from build123d import *

# Parameters (mm, degrees)
CHAMFER1_SIZE       = 1
SKETCH2_R           = 2.5
BOSS_EXTRUDE1_DEPTH = 1


with BuildPart() as part:
    # Sketch1 → Revolve1 (revolve)
    with BuildSketch(Plane.XY, mode=Mode.PRIVATE) as revolve1_sk:
        Polygon((0, 25), (-5, 25), (-5, 23), (-2.5, 23), (-2.5, 22), (-2, 22), (-2, 0), (-0.45, 0), (-0.45, 19), (0, 19), align=None)
    revolve(revolve1_sk.sketch.rotate(Axis((0, 0, 0), (0, 1, 0)), 270), axis=Axis((0, 0, 0), (0, 1, 0)))

    # Chamfer1
    chamfer1_edges = [part.edges().sort_by_distance(p)[0] for p in [
        (0, 0, 2),
    ]]
    chamfer(chamfer1_edges, length=CHAMFER1_SIZE)

    # Sketch2 → Boss-Extrude1 (add)
    with BuildSketch(Plane(origin=(0, 25, 0), x_dir=(1, 0, 0), z_dir=(0, 1, 0))):
        with Locations(Location((0, 0, 0), (0, 0, 90))):
            Circle(SKETCH2_R)
    extrude(amount=BOSS_EXTRUDE1_DEPTH)


solid = part.part
Here's how the part is built. I have some questions about the finished solid (model axes, mm). A direction names the side the tool comes from. Coordinates: 2 decimals unless noted, no trailing zeros. Write each loop counter-clockwise with the first axis right and the second up, starting at its lowest first coordinate (ties: lowest second). Pieces come first, ordered by that corner, then holes.
1) If I drill on line 1 (X direction, y = 13, z = 0); line 2 (Y direction, x = 1.5, z = 3); line 3 (Z direction, x = 0.25, y = 11.75), over which ranges is the centre line in solid material (lowest first)?
Filled in:
line 1: x = -2 to -0.45, 0.45 to 2
line 2: y = 23 to 25
line 3: z = -1.98 to -0.37, 0.37 to 1.98
2) If we section it at A-A (x = 0): List the corners of the cut face in (y, z) for me.
Filled in:
outline: (0, -1) - (1, -2) - (22, -2) - (22, -2.5) - (23, -2.5) - (23, -5) - (25, -5) - (25, -2.5) - (26, -2.5) - (26, 2.5) - (25, 2.5) - (25, 5) - (23, 5) - (23, 2.5) - (22, 2.5) - (22, 2) - (1, 2) - (0, 1) - (0, 0.45) - (19, 0.45) - (19, -0.45) - (0, -0.45) - close
3) If we section it at B-B (y = 2.25): List the corners of the cut face in (x, z) for me, plus the area to 3 significant figures.
Filled in:
outline: circle Ø4 at (0, 0); hole circle Ø0.9 at (0, 0)
area: 11.9 mm2
4) Thinking about a two-plate mould opening in X: for faces 3 (the face through (0, 26, 0)), 4 (the face through (0.172, 9.633, -0.416)), 5 (the face through (4.88, 23.99, 1.08)), which applies, +X half, -X half, draft (parallel to the pull), parting line (faces both ways), or undercut?
Filled in:
face 3: draft
face 4: undercut
face 5: parting line
5) I'm going to push flat-ended pins straight in: pin 1 (1.5 mm diameter, centred on x = -1, z = -3.5, fed in from -Y); pin 2 (6 mm diameter, centred on y = 7, z = 3, fed in from +X); pin 3 (3 mm diameter, centred on y = 15, z = -4, fed in from +X); pin 4 (4 mm diameter, centred on x = -1, y = 7, fed in from +Z). Where does each tip first touch, or does it pass through?
Filled in:
pin 1: stops at y = 23
pin 2: stops at x = 2
pin 3: passes through
pin 4: stops at z = 2
6) If we section it at C-C (z = 0): List the corners of the cut face in (x, y) for me.
Filled in:
outline: (-5, 23) - (-2.5, 23) - (-2.5, 22) - (-2, 22) - (-2, 1) - (-1, 0) - (-0.45, 0) - (-0.45, 19) - (0.45, 19) - (0.45, 0) - (1, 0) - (2, 1) - (2, 22) - (2.5, 22) - (2.5, 23) - (5, 23) - (5, 25) - (2.5, 25) - (2.5, 26) - (-2.5, 26) - (-2.5, 25) - (-5, 25) - close
7) If we section it at D-D (y = 24): List the corners of the cut face in (x, z) for me.
Filled in:
outline: circle Ø10 at (0, 0)
8) Which directions (+Z, -Z, +X, -X, +Y, -Y) give clear straight access to the entire face, cutting with the end or side of a thin tool? Please do faces 1 (the face through (2, 25, 2)), 2 (the face through (-2, 22, 1)).
Filled in:
face 1: +Y
face 2: -Y
